The model under review builds one solid part; all positions refer to its coordinate system, in mm. Face numbers are marked on the shaded views. A direction names the side the tool comes from. Coordinates: 2 decimals unless noted, no trailing zeros. Order: outer loops, then holes, each group sorted by start corner. A loop starts at its lowest first (then second) coordinate and runs counter-clockwise, first axis right, second up.
```python
from build123d import *

# Parameters (mm, degrees)
SKETCH1_R           = 6
SKETCH1_R_2         = 2.75
BOSS_EXTRUDE1_DEPTH = 8
SKETCH2_R           = 11.25
CUT_EXTRUDE1_DEPTH  = 3.2


with BuildPart() as part:
    # Sketch1 → Boss-Extrude1 (new body)
    with BuildSketch(Plane(origin=(0, 0, 0), x_dir=(1, 0, 0), z_dir=(0, 1, 0))):
        with BuildLine():
            Line((-12.990381057, 13), (12.990381057, 13))
            ThreePointArc((12.990381057, 13), (17.753520778, 10.25), (17.753520778, 4.75))
            Line((17.753520778, 4.75), (4.763139721, -17.75))
            ThreePointArc((4.763139721, -17.75), (0, -20.5), (-4.763139721, -17.75))
            Line((-4.763139721, -17.75), (-17.753520778, 4.75))
            ThreePointArc((-17.753520778, 4.75), (-17.753520778, 10.25), (-12.990381057, 13))
        make_face()
        Circle(SKETCH1_R, mode=Mode.SUBTRACT)
        with Locations((-12.990381057, 7.5)):
            Circle(SKETCH1_R_2, mode=Mode.SUBTRACT)
        with Locations((12.990381057, 7.5)):
            Circle(SKETCH1_R_2, mode=Mode.SUBTRACT)
        with Locations((0, -15)):
            Circle(SKETCH1_R_2, mode=Mode.SUBTRACT)
    extrude(amount=BOSS_EXTRUDE1_DEPTH)

    # Sketch2 → Cut-Extrude1 (cut)
    with BuildSketch(Plane.XZ):
        Circle(SKETCH2_R)
    extrude(amount=-CUT_EXTRUDE1_DEPTH, mode=Mode.SUBTRACT)


solid = part.part
```
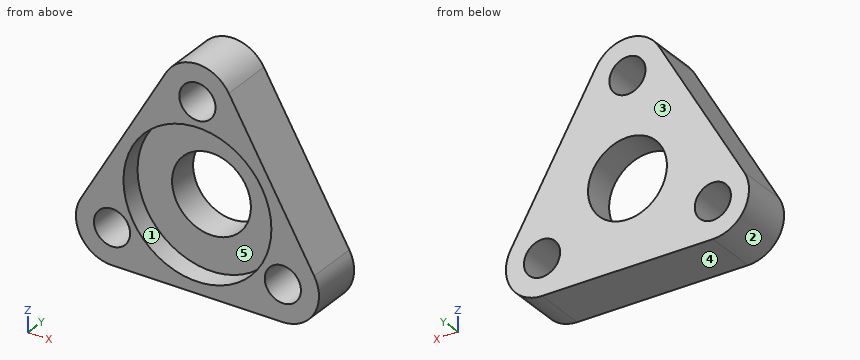
(1) Wall thickness on probe 1 along Z at (x, y) = (0, 1.35); probe 2 along X at (y, z) = (3.75, -7.5); probe 3 along Z at (x, y) = (0, 6.25): over which ranges is each line inside the solid? List them lowest first.
A:
probe 1: z = -13 to -11.25, 11.25 to 12.25, 17.75 to 20.5
probe 2: x = -18.49 to -15.74, -10.24 to 10.24, 15.74 to 18.49
probe 3: z = -13 to -6, 6 to 12.25, 17.75 to 20.5
(2) Machinability: for the marked faces 4 and 5, which of the approach directions +Z, -Z, +X, -X, +Y, -Y give a long, thin tool a straight path to every point of the face, cutting with its end or side? Answer none if there is none.
A:
face 4: -Z, +X, -X, +Y, -Y
face 5: -Y
(3) We need section C-C, the plane y = 5.25. Write out the cut boundary in (x, z), and give its area (3 significant figures).
A:
outline: (-17.75, -4.75) arc R5.5 ccw to (-12.99, -13) - (12.99, -13) arc R5.5 ccw to (17.75, -4.75) - (4.76, 17.75) arc R5.5 ccw to (-4.76, 17.75) - close; hole circle Ø5.5 at (-12.99, -7.5); hole circle Ø12 at (0, 0); hole circle Ø5.5 at (0, 15); hole circle Ø5.5 at (12.99, -7.5)
area: 632 mm2
(4) We need section A-A, the plane x = 0. Write out the cut boundary in (y, z).
A:
outline: (0, -13) - (8, -13) - (8, -6) - (3.2, -6) - (3.2, -11.25) - (0, -11.25) - close; (0, 11.25) - (3.2, 11.25) - (3.2, 6) - (8, 6) - (8, 12.25) - (0, 12.25) - close; (0, 17.75) - (8, 17.75) - (8, 20.5) - (0, 20.5) - close
(5) For pin 1 Ø1.5 at (y, z) = (2, 4.5) entering from -X; pin 2 Ø9 at (x, z) = (0, 15) entering from +Y; pin 3 Ø2 at (y, z) = (3, -5) entering from -X; pin 4 Ø1.5 at (x, y) = (13, 6.5) entering from +Z, all flat-tipped, find the tip position at first contact; note any pin that passes through.
A:
pin 1: stops at x = -12.85
pin 2: stops at y = 8
pin 3: stops at x = -18.28
pin 4: stops at z = 4.78
(6) Draft analysis for pull direction X (two halves, no side actions). For the marked faces 1, 2 and 3, state which applies: released by +X, released by -X, zero draft, split by the parting line, or undercut.
A:
face 1: undercut
face 2: released by -X
face 3: zero draft
(7) We need section D-D, the plane z = 0. Write out the cut boundary in (x, y).
A:
outline: (-15.01, 0) - (-11.25, 0) - (-11.25, 3.2) - (-6, 3.2) - (-6, 8) - (-15.01, 8) - close; (6, 3.2) - (11.25, 3.2) - (11.25, 0) - (15.01, 0) - (15.01, 8) - (6, 8) - close
(8) We need section B-B, the plane z = -7.5. Write out the cut boundary in (x, y).
A:
outline: (-18.49, 0) - (-15.74, 0) - (-15.74, 8) - (-18.49, 8) - close; (-10.24, 0) - (-8.39, 0) - (-8.39, 3.2) - (8.39, 3.2) - (8.39, 0) - (10.24, 0) - (10.24, 8) - (-10.24, 8) - close; (15.74, 0) - (18.49, 0) - (18.49, 8) - (15.74, 8) - close
